Source: CAD feature listing. Evaluate the final solid. Frame: model axes, mm. Face numbers are marked on the shaded views. Round coordinates to 2 decimals unless told otherwise and drop trailing zeros. Order: outer loops, then holes, each group sorted by start corner. A loop starts at its lowest first (then second) coordinate and runs counter-clockwise, first axis right, second up. Notation, with made-up numbers: M -12.75,88 L 26.25,88 A9 ccw 26.25,102 Z; hole C 39,50 d6. An arc over 180 degrees is marked long. Answer in a Markdown table with one row per item. Add a question column.
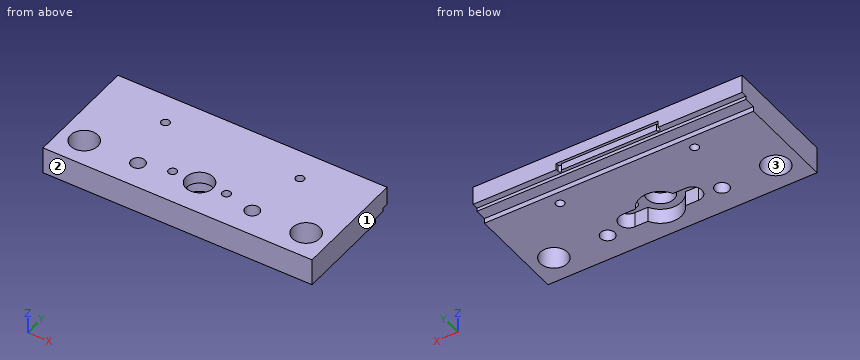
```python
from build123d import *

# Parameters (mm, degrees)
SKETCH_2_W           = 80
SKETCH_2_H           = 34
SKETCH_2_R           = 4.05
EXTRUDE_1_DEPTH      = 8
CUT_EXTRUDE_2_DEPTH  = 88.292611371
CUT_EXTRUDE_12_DEPTH = 4.5
SKETCH_20_R          = 6.25
CUT_EXTRUDE_13_DEPTH = 4.5
CUT_EXTRUDE_11_DEPTH = 2
HOLE_WIZARD_M3_7_D   = 2.5
HOLE_WIZARD_M5_1_D   = 4.2


with BuildPart() as part:
    # 草图2 → 凸台-拉伸1 (new body)
    with BuildSketch(Plane.XY):
        with Locations((40, 17)):
            Rectangle(SKETCH_2_W, SKETCH_2_H)
        with Locations((7, 8)):
            Circle(SKETCH_2_R, mode=Mode.SUBTRACT)
        with Locations((40, 10)):
            Circle(SKETCH_2_R, mode=Mode.SUBTRACT)
        with Locations((73, 8)):
            Circle(SKETCH_2_R, mode=Mode.SUBTRACT)
    extrude(amount=EXTRUDE_1_DEPTH)

    # 草图4 → 切除-拉伸2 (cut, through all)
    with BuildSketch(Plane(origin=(80, 0, 0), x_dir=(0, 0, -1), z_dir=(1, 0, 0))):
        Polygon((-1.5, 32.2), (-2.5, 32.2), (-2.5, 34), (0, 34), (0, 28.8), (-1.5, 28.8), align=None)
    extrude(amount=-CUT_EXTRUDE_2_DEPTH, mode=Mode.SUBTRACT)

    # 草图8 → 切除-拉伸12 (cut)
    with BuildSketch(Plane(origin=(0, 0, 0), x_dir=(-1, 0, 0), z_dir=(0, 0, -1))):
        with BuildLine():
            Line((-30.5, 12.85), (-49.5, 12.85))
            ThreePointArc((-49.5, 12.85), (-52.35, 10), (-49.5, 7.15))
            Line((-49.5, 7.15), (-30.5, 7.15))
            ThreePointArc((-30.5, 7.15), (-27.65, 10), (-30.5, 12.85))
        make_face()
    extrude(amount=-CUT_EXTRUDE_12_DEPTH, mode=Mode.SUBTRACT)

    # 草图20 → 切除-拉伸13 (cut)
    with BuildSketch(Plane(origin=(0, 0, 0), x_dir=(-1, 0, 0), z_dir=(0, 0, -1))):
        with Locations((-40, 10)):
            Circle(SKETCH_20_R)
    extrude(amount=-CUT_EXTRUDE_13_DEPTH, mode=Mode.SUBTRACT)

    # 草图19 → 切除-拉伸11 (cut)
    with BuildSketch(Plane(origin=(0, 0, 2.5), x_dir=(-1, 0, 0), z_dir=(0, 0, -1))):
        with BuildLine():
            Line((-25, 34), (-55.247938178, 34))
            Line((-55.247938178, 34), (-55.247938178, 33.2))
            ThreePointArc((-55.247938178, 33.2), (-54.747938178, 32.7), (-54.247938178, 33.2))
            Line((-54.247938178, 33.2), (-26, 33.2))
            ThreePointArc((-26, 33.2), (-25.5, 32.7), (-25, 33.2))
            Line((-25, 33.2), (-25, 34))
        make_face()
    extrude(amount=-CUT_EXTRUDE_11_DEPTH, mode=Mode.SUBTRACT)

    # M3 螺纹孔7 (through all)
    with Locations(Plane.XY.offset(8)):
        with Locations((20, 25), (60, 25), (32, 10), (48, 10)):
            Hole(HOLE_WIZARD_M3_7_D / 2)

    # M5 螺纹孔1 (through all)
    with Locations(Plane.XY.offset(8)):
        with Locations((23, 8), (57, 8)):
            Hole(HOLE_WIZARD_M5_1_D / 2)


solid = part.part
```
(1) Draft query along Y for the marked faces 1, 2 and 3. Return one class per face: +Y half, -Y half, draft (parallel to the pull), parting line (faces both ways), or undercut.
(2) Pin query (flat end, axial travel): pin 1 (4 mm diameter, centred on x = 37.5, y = 10.5, fed in from -Z); pin 2 (3 mm diameter, centred on x = 31.5, z = 1.5, fed in from +Y); pin 3 (1.4 mm diameter, centred on x = 50, y = 33.5, fed in from -Z). Return the tip coordinate at first contact, or that it passes through.
(3) Line query: line 1 (X direction, y = 11.5, z = 3); line 2 (Y direction, x = 73, z = 1.75); line 3 (Z direction, x = 68, y = 29.5). Output: solid intervals per line, ascending. Write a range as from..to.
(4) Cut plane D-D (x = 23). Return loops of the section in (y, z), and give its area (3 significant figures).
(5) Cut plane A-A (x = 40). Return loops of the section in (y, z).
(6) Cut plane B-B (z = 5.25). Count the separate pieces of the cut face and the enclosed holes in it, and give its area (3 significant figures).
(7) Cut plane C-C (x = 48). Return loops of the section in (y, z).
Answer list:
| question | item | result |
|---|---|---|
| 1 | face 1 | draft |
| 1 | face 2 | -Y half |
| 1 | face 3 | undercut |
| 2 | pin 1 | z = 4.5 |
| 2 | pin 2 | y = 33.2 |
| 2 | pin 3 | z = 2.5 |
| 3 | line 1 | 0..4.96, 9.04..28.08, 51.92..70.96, 75.04..80 |
| 3 | line 2 | 0..3.95, 12.05..32.2 |
| 3 | line 3 | 1.5..8 |
| 4 | outline | M 0,0 L 5.9,0 L 5.9,8 L 0,8 Z; M 10.1,0 L 28.8,0 L 28.8,1.5 L 32.2,1.5 L 32.2,2.5 L 34,2.5 L 34,8 L 10.1,8 Z |
| 4 | area | 229 mm² |
| 5 | outline | M 0,0 L 3.75,0 L 3.75,4.5 L 5.95,4.5 L 5.95,8 L 0,8 Z; M 14.05,4.5 L 16.25,4.5 L 16.25,0 L 28.8,0 L 28.8,1.5 L 32.2,1.5 L 32.2,2.5 L 33.2,2.5 L 33.2,4.5 L 34,4.5 L 34,8 L 14.05,8 Z |
| 6 | separate pieces | 1 |
| 6 | enclosed holes | 9 |
| 6 | area | 2,520 mm² |
| 7 | outline | M 0,0 L 7.15,0 L 7.15,4.5 L 8.75,4.5 L 8.75,8 L 0,8 Z; M 11.25,4.5 L 12.85,4.5 L 12.85,0 L 28.8,0 L 28.8,1.5 L 32.2,1.5 L 32.2,2.5 L 33.2,2.5 L 33.2,4.5 L 34,4.5 L 34,8 L 11.25,8 Z |
